Autodesk Inventor part; units mm, degrees
ref_plane "YZ Plane" through (0, 0, 0) normal (1, 0, 0) x (0, 1, 0)
ref_plane "XZ Plane" through (0, 0, 0) normal (0, 1, 0) x (-1, 0, 0)
ref_plane "XY Plane" through (0, 0, 0) normal (0, 0, 1) x (1, 0, 0)
sketch "Sketch1" plane through (0, 0, 0) normal (0, 1, 0) x (-1, 0, 0)
  circle A0 centre (49.0175, 1.0065) radius 3.6
  line L0 (58.9307, -3.2235) -> (48.4307, -3.2235)
  line L1 (58.9307, -3.2235) -> (58.9307, 22.7221)
  line L2 (58.9307, 22.7221) -> (56.4307, 22.7221)
  line L3 (56.4307, 22.7221) -> (53.9307, 7.6757)
  line L4 (53.9307, 7.6757) -> (53.9307, 4.6065)
  line L5 (53.9307, 4.6065) -> (49.0175, 4.6065)
  line L6 (53.4307, -3.2235) -> (53.4307, 4.6065)
  line L7 (46.6824, -1.7334) -> (48.4307, -3.2235)
  circle A1 centre (49.0175, 1.0065) radius 3
  point P0 (0, 0)
  dimension "d0" = 5.5
  dimension "d1" = 5
  dimension "d2" = 2.5
  dimension "d3" = 10.5
  dimension "d4" = 7.2
  dimension "d5" = 6
  dimension "d14" = 4.23
extrude "Extrusion1" add sketch "Sketch1" along normal mid plane 4.1
extrude "Extrusion2" add sketch "Sketch1" along normal mid plane 12 contours L5 L4 L3 L2 L1 L0 L6
fillet "Fillet1" radius 2 3 edges at (-56.4307, 0, 22.7221) (-55.1807, 6, 15.1989) (-55.1807, -6, 15.1989)
chamfer "Chamfer1" distance 2 angle 45 1 edges at (-58.9307, 0, -3.2235)
properties part number "Foot"
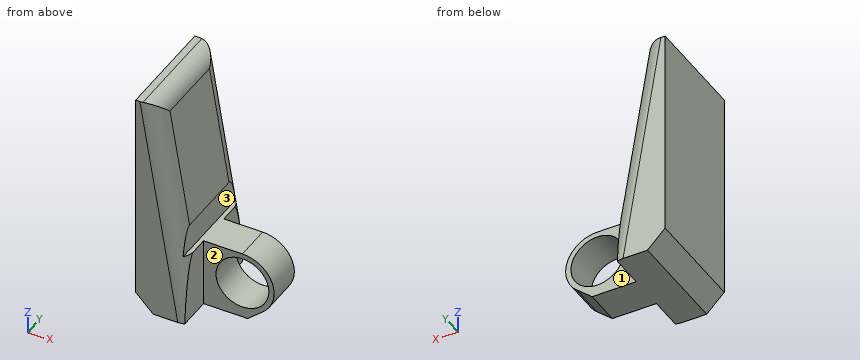
Input: part model. Units: mm. Frame: model coordinates. Face numbers are marked on the shaded views. A direction names the side the tool comes from. Coordinates: 2 decimals unless noted, no trailing zeros. Order: outer loops, then holes, each group sorted by start corner. A loop starts at its lowest first (then second) coordinate and runs counter-clockwise, first axis right, second up. Notation, with made-up numbers: (39.25, 0.5) - (59.25, 0.5) arc R6 cw to (59.25, 7.5) - close; hole circle Ø10 at (-36.5, 54). An arc over 180 degrees is marked (long way). Put each result on its own line as item: value.
1. Contact query for flat-ended pins moving along their axis: pin 1 Ø5.5 at (x, y) = (-50.5, 2) entering from +Z; pin 2 Ø4 at (y, z) = (3, 1.5) entering from +X; pin 3 Ø1.1 at (y, z) = (-3, 2.5) entering from +X; pin 4 Ø1.5 at (x, y) = (-47, -0.5) entering from +Z. Output: stop coordinate, or through.
Report:
pin 1: stops at z = 4.61
pin 2: stops at x = -45.42
pin 3: stops at x = -53.43
pin 4: stops at z = 4.38
2. Cut plane A-A on x = -47.75. Return the cut outline in (y, z), then the cut area to 3 significant figures.
Report:
outline: (-2.05, -2.64) - (2.05, -2.64) - (2.05, -1.71) - (-2.05, -1.71) - close; (-2.05, 3.73) - (2.05, 3.73) - (2.05, 4.38) - (-2.05, 4.38) - close
area: 6.48 mm2
3. Reachability of the marked faces 1, 2 and 3 from +Z, -Z, +X, -X, +Y, -Y: full face, straight path, thin tool, end or side. Return the list, or none.
Report:
face 1: +Z, -Z, +X, +Y
face 2: +Z, -Z, +X, -Y
face 3: +Z, +X, +Y, -Y
4. Cut plane C-C on y = -5. Return the cut outline in (x, z), then the cut area to 3 significant figures.
Report:
outline: (-58.93, -1.22) - (-56.93, -3.22) - (-53.43, -3.22) - (-53.43, 3.03) - (-53.69, 4.61) - (-53.93, 4.61) - (-53.93, 6.04) - (-56.58, 21.99) arc R2 ccw to (-58.13, 22.72) - (-58.93, 22.72) - close
area: 108 mm2
5. Line query: line 1 along X through (y, z) = (4.5, 1.75); line 2 along Z through (x, y) = (-50, 0.5); line 3 along X through (y, z) = (-3, 5.5). Output: solid intervals per line, ascending.
Report:
line 1: x = -58.93 to -53.43
line 2: z = -3.22 to -1.83, 3.84 to 4.61
line 3: x = -58.93 to -53.93
6. Cut plane B-B on y = -1.75. Return the cut outline in (x, z).
Report:
outline: (-58.93, -1.22) - (-56.93, -3.22) - (-48.43, -3.22) - (-46.68, -1.73) arc R3.6 ccw to (-49.02, 4.61) - (-53.93, 4.61) - (-53.93, 7.68) - (-56.15, 21.05) arc R2 ccw to (-58.13, 22.72) - (-58.93, 22.72) - close; hole circle Ø6 at (-49.02, 1.01)
7. Cut plane D-D on x = -52.75. Return the cut outline in (y, z), then the cut area to 3 significant figures.
Report:
outline: (-2.05, -3.22) - (2.05, -3.22) - (2.05, 4.61) - (-2.05, 4.61) - close
area: 32.1 mm2
